CAD build for the part. Positions are in the model's coordinates, mm. A direction names the side the tool comes from. Round coordinates to 2 decimals unless told otherwise and drop trailing zeros. Order: outer loops, then holes, each group sorted by start corner. A loop starts at its lowest first (then second) coordinate and runs counter-clockwise, first axis right, second up. Notation, with made-up numbers: M 71.5,33 L 83.5,33 A25 cw 83.5,60 Z; hole C -19.5,16.5 d3. An arc over 180 degrees is marked long. Answer as a JSON object with one key per item and string values. Group by question number.
```python
from build123d import *

# Parameters (mm, degrees)
SKETCH_1_W          = 40
SKETCH_1_H          = 40
EXTRUDE_1_DEPTH     = 20
SKETCH_2_R          = 3
EXTRUDE_2_DEPTH     = 6
EXTRUDE_START       = -8
SKETCH_3_W          = 20
SKETCH_3_H          = 7.5
EXTRUDE_3_DEPTH     = 3
SKETCH_4_R          = 2.25
CUT_EXTRUDE_1_DEPTH = 3
FILLET_1_R          = 0.5


with BuildPart() as part:
    # 草图1 → 凸台-拉伸1 (new body)
    with BuildSketch(Plane(origin=(0, 0, 0), x_dir=(0, 0, -1), z_dir=(1, 0, 0))):
        Rectangle(SKETCH_1_W, SKETCH_1_H)
    extrude(amount=EXTRUDE_1_DEPTH)

    # 草图2 → 凸台-拉伸2 (add)
    with BuildSketch(Plane(origin=(0, 20, 0), x_dir=(1, 0, 0), z_dir=(0, 1, 0))):
        with Locations(Location((10, -10, 0), (0, 0, 90))):
            Circle(SKETCH_2_R)
    extrude(amount=EXTRUDE_2_DEPTH)

    # 草图3 → 凸台-拉伸3 (add)
    with BuildSketch(Plane(origin=(0, 20, 0), x_dir=(1, 0, 0), z_dir=(0, 1, 0)).offset(EXTRUDE_START)):
        with Locations((10, -23.75)):
            Rectangle(SKETCH_3_W, SKETCH_3_H)
        with Locations((10, 23.75)):
            Rectangle(SKETCH_3_W, SKETCH_3_H)
    extrude(amount=-EXTRUDE_3_DEPTH)

    # 草图4 → 切除-拉伸1 (cut)
    with BuildSketch(Plane(origin=(0, 12, 0), x_dir=(1, 0, 0), z_dir=(0, 1, 0))):
        with Locations(Location((14.5, -24.5, 0), (0, 0, 270))):
            Circle(SKETCH_4_R)
        with Locations(Location((5.5, -24.5, 0), (0, 0, 270))):
            Circle(SKETCH_4_R)
        with Locations(Location((5.5, 24.5, 0), (0, 0, 90))):
            Circle(SKETCH_4_R)
        with Locations(Location((14.5, 24.5, 0), (0, 0, 90))):
            Circle(SKETCH_4_R)
    extrude(amount=-CUT_EXTRUDE_1_DEPTH, mode=Mode.SUBTRACT)

    # 圆角1
    fillet_1_edges = [part.edges().sort_by_distance(p)[0] for p in [
        (20, -5.5, -20),
        (20, 20, 0),
        (0, 16, -20),
        (20, 16, -20),
        (0, -5.5, 20),
        (20, -5.5, 20),
        (0, 9, 23.75),
        (0, 10.5, 27.5),
        (20, 9, 23.75),
        (20, 10.5, 27.5),
        (0, 12, 23.75),
        (20, 12, 23.75),
        (0, 9, -23.75),
        (0, 10.5, -27.5),
        (20, 9, -23.75),
        (20, 10.5, -27.5),
        (0, 12, -23.75),
        (20, 12, -23.75),
        (20, 16, 20),
        (0, 20, 0),
        (0, -5.5, -20),
        (0, -20, 0),
        (0, 16, 20),
        (20, -20, 0),
    ]]
    fillet(fillet_1_edges, radius=FILLET_1_R)


solid = part.part
```
Item 1: Two-plate mould, pull along X, no slides. Class faces 1 (the face through (10, -20, 0)), 2 (the face through (4.824, 10.521, -26.646)), 3 (the face through (0, 0, 0)), 4 (the face through (13.824, 10.521, -26.646)): +X half, -X half, draft (parallel to the pull), parting line (faces both ways), or undercut.
Item 2: Drill centre lines: line 1 (X direction, y = 10.95, z = -24.5); line 2 (Y direction, x = 13.5, z = -18.5). Where is each one in solid material? Low to high. Write a range as [from, to].
Item 3: 3-axis set-ups, long thin cutter, end or side, ignore diameter. For faces 5 (the face through (7.97, 22.96, 12.21)), 6 (the face through (10, 9, 24)), 7 (the face through (10, 16, -20)), 8 (the face through (10, -6, -20)): which of +Z, -Z, +X, -X, +Y, -Y reach the whole face in a straight line?
Item 4: Cut at C-C, the plane y = -4. Give the cut face in (x, z).
Item 5: Cut at A-A, the plane z = 24.5. Give the cut face in (x, y).
Item 6: Cut at B-B, the plane x = 14.5. Give the cut face in (y, z), and give its area (3 significant figures).
Item 7: Cut at D-D, the plane x = 10. Give the cut face in (y, z).
Item 8: Flat gauge pins, fed straight in: pin 1 Ø8 at (x, z) = (13, 25) entering from +Y; pin 2 Ø2.5 at (x, z) = (5.5, -24.5) entering from -Y; pin 3 Ø10 at (x, z) = (7.5, -16) entering from +Y; pin 4 Ø7 at (x, z) = (14.5, -24.5) entering from -Y. Where does each tip first touch, or does it go through?
Response values:
{
 "1": {"face 1": "draft", "face 2": "undercut", "face 3": "-X half", "face 4": "undercut"},
 "2": {"line 1": "[0, 3.25], [7.75, 12.25], [16.75, 20]", "line 2": "[-20, 20]"},
 "3": {"face 5": "+Y", "face 6": "+Z, +X, -X, -Y", "face 7": "-Z, +X, -X, +Y", "face 8": "-Z, +X, -X, -Y"},
 "4": {"outline": "M 0,-19.5 A0.5 ccw 0.5,-20 L 19.5,-20 A0.5 ccw 20,-19.5 L 20,19.5 A0.5 ccw 19.5,20 L 0.5,20 A0.5 ccw 0,19.5 Z"},
 "5": {"outline": "M 0,9.5 A0.5 ccw 0.5,9 L 3.25,9 L 3.25,12 L 0.5,12 A0.5 ccw 0,11.5 Z; M 7.75,9 L 12.25,9 L 12.25,12 L 7.75,12 Z; M 16.75,9 L 19.5,9 A0.5 ccw 20,9.5 L 20,11.5 A0.5 ccw 19.5,12 L 16.75,12 Z"},
 "6": {"outline": "M -20,-20 L 9,-20 L 9,-22.25 L 12,-22.25 L 12,-20 L 20,-20 L 20,20 L 12,20 L 12,22.25 L 9,22.25 L 9,20 L -20,20 Z; M 9,-27.5 L 12,-27.5 L 12,-26.75 L 9,-26.75 Z; M 9,26.75 L 12,26.75 L 12,27.5 L 9,27.5 Z", "area": "1,620 mm^2"},
 "7": {"outline": "M -20,-20 L 9,-20 L 9,-27.5 L 12,-27.5 L 12,-20 L 20,-20 L 20,7 L 26,7 L 26,13 L 20,13 L 20,20 L 12,20 L 12,27.5 L 9,27.5 L 9,20 L -20,20 Z"},
 "8": {"pin 1": "y = 12", "pin 2": "through", "pin 3": "y = 20", "pin 4": "y = 9"}
}
